```python
from build123d import *

# Parameters (mm, degrees)
F0_R     = 3.913222
F0_R_2   = 1.012094
F0_R_3   = 3.607223
F1_DEPTH = 5


with BuildPart() as f1:
    # F0 (on Top) → F1 (new body)
    with BuildSketch(Plane.XY):
        with BuildLine():
            ThreePointArc((-23.629729, 22.588529), (-24.336836, 22.295636), (-24.629729, 21.588529))
            Line((-24.629729, 21.588529), (-24.629729, -2.411471))
            Line((-24.629729, -2.411471), (-16.771118, -2.411471))
            ThreePointArc((-16.771118, -2.411471), (-10.089518, 3.50554), (-15.155087, 10.853656))
            ThreePointArc((-15.155087, 10.853656), (-11.437269, 18.035431), (-18.120783, 22.588529))
            Line((-18.120783, 22.588529), (-23.629729, 22.588529))
        make_face()
        with Locations((-16.771118, 4.319529)):
            Circle(F0_R, mode=Mode.SUBTRACT)
        with Locations((-22.511555, 20.511821)):
            Circle(F0_R_2, mode=Mode.SUBTRACT)
        with Locations((-17.347449, 16.541781)):
            Circle(F0_R_3, mode=Mode.SUBTRACT)
    extrude(amount=F1_DEPTH)


solid = f1.part
```
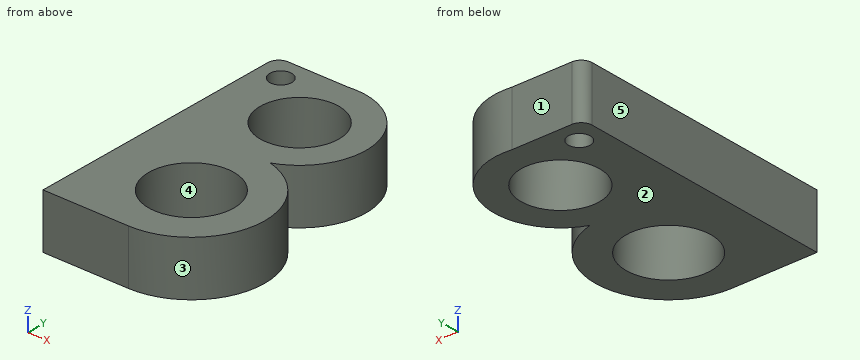
For this review, take the finished solid that the model builds, in its own axes (mm). Face numbers are marked on the shaded views. A direction names the side the tool comes from. Round coordinates to 2 decimals unless told otherwise and drop trailing zeros. Loops run counter-clockwise (first coordinate to the right, second up) from the corner with the lowest first, then second, coordinate; pieces in that order, holes last.
(1) Mouldability with a two-part tool opening along X and no side actions: class the marked faces 3, 4 and 5 as released by +X, released by -X, zero draft, split by the parting line, or undercut.
Returned:
face 3: released by +X
face 4: undercut
face 5: released by -X
(2) Wall thickness on line 1 along Y through (x, z) = (-16.5, 4); line 2 along Y through (x, z) = (-18, 4.35); line 3 along Y through (x, z) = (-21, 2.45): over which ranges is each line inside the solid? List them lowest first.
Returned:
line 1: y = -2.41 to 0.42, 8.22 to 13.04, 20.05 to 22.58
line 2: y = -2.41 to 0.6, 8.03 to 12.99, 20.09 to 22.6
line 3: y = -2.41 to 22.59
(3) Clearance check with flat-ended pins moving along their axes: P1, Ø1.5, axis at x = -15, z = 2.5, coming from the -Y side; P2, Ø1, axis at y = 12, z = 4.5, coming from the +X side; P3, Ø1, axis at y = 1, z = 4.5, coming from the +X side. State where each tip first meets the part, or that it passes through.
Returned:
P1: stops at y = -2.33
P2: stops at x = -12.78
P3: stops at x = -10.66
(4) We need section C-C (x = -16.5). Give the boundary of the cut face in (y, z).
Returned:
outline: (-2.41, 0) - (0.42, 0) - (0.42, 5) - (-2.41, 5) - close; (8.22, 0) - (13.04, 0) - (13.04, 5) - (8.22, 5) - close; (20.05, 0) - (22.58, 0) - (22.58, 5) - (20.05, 5) - close
(5) Tool access review of the marked faces 1 and 2: name each direction out of +Z, -Z, +X, -X, +Y, -Y from which nothing blocks a thin tool from reaching the whole face with its end or side.
Returned:
face 1: +Z, -Z, -X, +Y
face 2: -Z, +X, -X, +Y, -Y
(6) We need section A-A (x = -23.25). Give the boundary of the cut face in (y, z).
Returned:
outline: (-2.41, 0) - (19.82, 0) - (19.82, 5) - (-2.41, 5) - close; (21.2, 0) - (22.59, 0) - (22.59, 5) - (21.2, 5) - close
(7) We need section B-B (y = 6). Give the boundary of the cut face in (x, z), plus the area to 3 significant figures.
Returned:
outline: (-24.63, 0) - (-20.31, 0) - (-20.31, 5) - (-24.63, 5) - close; (-13.24, 0) - (-10.25, 0) - (-10.25, 5) - (-13.24, 5) - close
area: 36.5 mm2
(8) We need section D-D (z = 3.6). Give the boundary of the cut face in (x, y), plus the area to 3 significant figures.
Returned:
outline: (-24.63, -2.41) - (-16.77, -2.41) arc R6.73 ccw to (-15.16, 10.85) arc R6.1 ccw to (-18.12, 22.59) - (-23.63, 22.59) arc R1 ccw to (-24.63, 21.59) - close; hole circle Ø2.02 at (-22.51, 20.51); hole circle Ø7.21 at (-17.35, 16.54); hole circle Ø7.83 at (-16.77, 4.32)
area: 226 mm2
